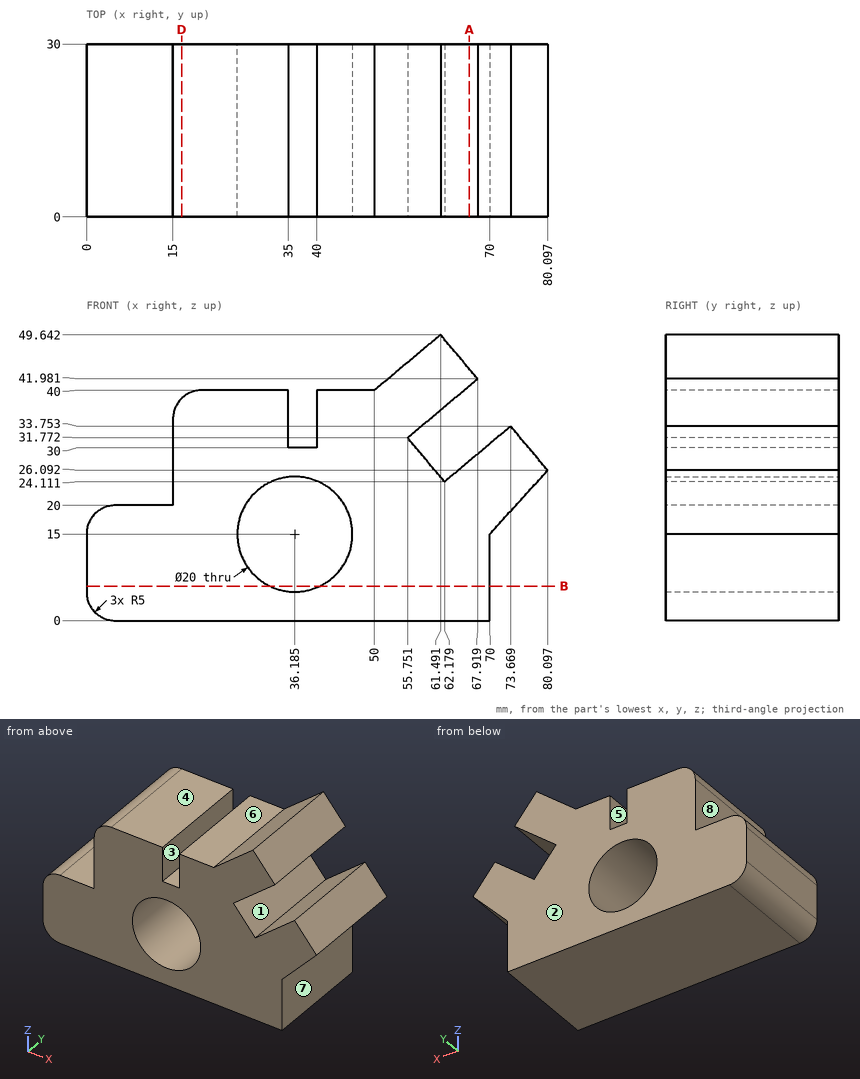
Source: three-view drawing plus pictorial views. Frame: mm from the lowest corner of the part. A direction names the side the tool comes from. Give positions to 0.01 mm unless a question says otherwise; leave off trailing zeros. Order: outer loops, then holes, each group sorted by start corner. A loop starts at its lowest first (then second) coordinate and runs counter-clockwise, first axis right, second up. Notation, with made-up numbers: (-19.75, 29.25) - (12.25, 29.25) arc R13 cw to (12.25, 54.25) - close; hole circle Ø1 at (86, -7.75). An arc over 180 degrees is marked (long way). Put each result on its own line as item: value.
Item 1: Draft query along X for the marked faces 5, 6, 7 and 8. Return one class per face: +X half, -X half, draft (parallel to the pull), parting line (faces both ways), or undercut.
Found:
face 5: undercut
face 6: draft
face 7: +X half
face 8: -X half
Item 2: Access query for the marked faces 1, 2, 3 and 4. Directions: +Z, -Z, +X, -X, +Y, -Y. A direction counts if a zero-diameter tool reaches every point of the face in a straight line with its end or side. Return the directions, or none.
Found:
face 1: +Y, -Y
face 2: +Z, -Z, +X, -X, +Y
face 3: +Z, +Y, -Y
face 4: +Z, -X, +Y, -Y
Item 3: Section query A-A, the plane x = 66.5. Return loops of the section in (y, z).
Found:
outline: (0, 0) - (30, 0) - (30, 27.74) - (0, 27.74) - close; (0, 40.79) - (30, 40.79) - (30, 43.67) - (0, 43.67) - close
Item 4: Section query B-B, the plane z = 6. Return loops of the section in (x, y), then the cut area to 3 significant figures.
Found:
outline: (0, 0) - (31.83, 0) - (31.83, 30) - (0, 30) - close; (40.54, 0) - (70, 0) - (70, 30) - (40.54, 30) - close
area: 1,840 mm^2
Item 5: Ray query, L1, parallel to X at y = 14.75, z = 33.5 (1 decimal); L2, parallel to X at y = 24.5, z = 31 (1 decimal); L3, parallel to Z at x = 14, y = 18. Return the intervals inside material, ascending. Write a range as from..to.
Found:
L1: x = 15..35, 40..57.8, 73.4..73.9
L2: x = 15..35, 40..56.4, 70.4..76
L3: z = 0..20
Item 6: Contact query for flat-ended pins moving along their axis: pin 1 (6 mm diameter, centred on y = 17.5, z = 20.5, fed in from +X); pin 2 (8 mm diameter, centred on x = 9, y = 15.5, fed in from +Z); pin 3 (8 mm diameter, centred on y = 17, z = 44.5, fed in from -X) (1 decimal); pin 4 (1.5 mm diameter, centred on x = 67.5, y = 18, fed in from -Z). Output: stop coordinate, or through.
Found:
pin 1: stops at x = 77.74
pin 2: stops at z = 20
pin 3: stops at x = 50.6
pin 4: stops at z = 0
Item 7: Section query D-D, the plane x = 16.5. Return loops of the section in (y, z), then the cut area to 3 significant figures.
Found:
outline: (0, 0) - (30, 0) - (30, 38.57) - (0, 38.57) - close
area: 1,160 mm^2
